```python
from build123d import *

# Parameters (mm, degrees)
ESQUISSE1_W                 = 200
ESQUISSE1_H                 = 200
BOSS_EXTRU_PAROIE_DEPTH     = 4
BOSS_EXTRU_BORDS_DEPTH      = 8
BOSS_EXTRU_GLISSIERES_DEPTH = 4
CONG_1_R                    = 1
ESQUISSE8_W                 = 1.8
ESQUISSE8_H                 = 180
ENL_V_MAT_EXTRU_6_DEPTH     = 9
ESQUISSE5_R                 = 1.6
ENL_V_MAT_EXTRU_2_DEPTH     = 10
ESQUISSE6_R                 = 1.6
ENL_V_MAT_EXTRU_3_DEPTH     = 10
ESQUISSE7_R                 = 1.6
ENL_V_MAT_EXTRU_4_DEPTH     = 10
ESQUISSE10_R                = 1.6
ENL_V_MAT_EXTRU_8_DEPTH     = 10
ESQUISSE11_W                = 113.303164178
ESQUISSE11_H                = 6
ENL_V_MAT_EXTRU_9_DEPTH     = 6
ESQUISSE9_R                 = 1.6
ENL_V_MAT_EXTRU_10_DEPTH    = 10


with BuildPart() as part:
    # Esquisse1 → Boss.-Extru. Paroie (new body)
    with BuildSketch(Plane.XY):
        with Locations((100, 100)):
            Rectangle(ESQUISSE1_W, ESQUISSE1_H)
    extrude(amount=BOSS_EXTRU_PAROIE_DEPTH)

    # Esquisse4 → Boss.-Extru. Bords (add)
    with BuildSketch(Plane.XY.offset(4)):
        Polygon((3, 3), (9, 3), (9, 184), (191, 184), (191, 3), (197, 3), (197, 197), (191, 197), (191, 190), (9, 190), (9, 197), (3, 197), align=None)
    extrude(amount=BOSS_EXTRU_BORDS_DEPTH)

    # Esquisse2 → Boss.-Extru. Glissieres (add)
    with BuildSketch(Plane.XY.offset(4)):
        with BuildLine():
            Line((47, 170), (53, 170))
            ThreePointArc((53, 170), (54.414213562, 169.414213562), (55, 168))
            Line((55, 168), (55, 32))
            ThreePointArc((55, 32), (54.414213562, 30.585786438), (53, 30))
            Line((53, 30), (47, 30))
            ThreePointArc((47, 30), (45.585786438, 30.585786438), (45, 32))
            Line((45, 32), (45, 168))
            ThreePointArc((45, 168), (45.585786438, 169.414213562), (47, 170))
        make_face()
        with BuildLine():
            Line((97, 170), (103, 170))
            ThreePointArc((103, 170), (104.414213562, 169.414213562), (105, 168))
            Line((105, 168), (105, 32))
            ThreePointArc((105, 32), (104.414213562, 30.585786438), (103, 30))
            Line((103, 30), (97, 30))
            ThreePointArc((97, 30), (95.585786438, 30.585786438), (95, 32))
            Line((95, 32), (95, 168))
            ThreePointArc((95, 168), (95.585786438, 169.414213562), (97, 170))
        make_face()
        with BuildLine():
            Line((147, 170), (153, 170))
            ThreePointArc((153, 170), (154.414213562, 169.414213562), (155, 168))
            Line((155, 168), (155, 32))
            ThreePointArc((155, 32), (154.414213562, 30.585786438), (153, 30))
            Line((153, 30), (147, 30))
            ThreePointArc((147, 30), (145.585786438, 30.585786438), (145, 32))
            Line((145, 32), (145, 168))
            ThreePointArc((145, 168), (145.585786438, 169.414213562), (147, 170))
        make_face()
    extrude(amount=BOSS_EXTRU_GLISSIERES_DEPTH)

    # Congé1
    cong_1_edges = [part.edges().sort_by_distance(p)[0] for p in [
        (200, 100, 4),
        (100, 200, 4),
        (0, 100, 4),
        (100, 0, 4),
    ]]
    fillet(cong_1_edges, radius=CONG_1_R)

    # Esquisse8 → Enlèv. mat.-Extru.6 (cut, through all)
    with BuildSketch(Plane.XY.offset(4)):
        with Locations((100, 85)):
            Rectangle(ESQUISSE8_W, ESQUISSE8_H)
        with Locations((150, 85)):
            Rectangle(ESQUISSE8_W, ESQUISSE8_H)
        with Locations((50, 85)):
            Rectangle(ESQUISSE8_W, ESQUISSE8_H)
    extrude(amount=ENL_V_MAT_EXTRU_6_DEPTH, mode=Mode.SUBTRACT)

    # Esquisse5 → Enlèv. mat.-Extru.2 (cut)
    with BuildSketch(Plane.ZY.offset(-3)):
        with Locations((8, 180)):
            Circle(ESQUISSE5_R)
        with Locations((8, 20)):
            Circle(ESQUISSE5_R)
    extrude(amount=-ENL_V_MAT_EXTRU_2_DEPTH, mode=Mode.SUBTRACT)

    # Esquisse6 → Enlèv. mat.-Extru.3 (cut)
    with BuildSketch(Plane(origin=(197, 0, 0), x_dir=(0, 0, -1), z_dir=(1, 0, 0))):
        with Locations((-8, 180)):
            Circle(ESQUISSE6_R)
        with Locations((-8, 20)):
            Circle(ESQUISSE6_R)
    extrude(amount=-ENL_V_MAT_EXTRU_3_DEPTH, mode=Mode.SUBTRACT)

    # Esquisse7 → Enlèv. mat.-Extru.4 (cut)
    with BuildSketch(Plane.XZ.offset(-184)):
        with Locations((35, 8)):
            Circle(ESQUISSE7_R)
        with Locations((165, 8)):
            Circle(ESQUISSE7_R)
    extrude(amount=-ENL_V_MAT_EXTRU_4_DEPTH, mode=Mode.SUBTRACT)

    # Esquisse10 → Enlèv. mat.-Extru.8 (cut)
    with BuildSketch(Plane(origin=(0, 3, 0), x_dir=(-1, 0, 0), z_dir=(0, -1, 0))):
        with Locations((-194.2, -8)):
            Circle(ESQUISSE10_R)
        with Locations((-5.8, -8)):
            Circle(ESQUISSE10_R)
    extrude(amount=-ENL_V_MAT_EXTRU_8_DEPTH, mode=Mode.SUBTRACT)

    # Esquisse11 → Enlèv. mat.-Extru.9 (cut)
    with BuildSketch(Plane.XY.offset(12)):
        with Locations((100.248809194, 187)):
            Rectangle(ESQUISSE11_W, ESQUISSE11_H)
    extrude(amount=-ENL_V_MAT_EXTRU_9_DEPTH, mode=Mode.SUBTRACT)

    # Esquisse9 → Enlèv. mat.-Extru.10 (cut)
    with BuildSketch(Plane(origin=(0, 197, 0), x_dir=(1, 0, 0), z_dir=(0, 1, 0))):
        with Locations((194.2, -8)):
            Circle(ESQUISSE9_R)
        with Locations((5.8, -8)):
            Circle(ESQUISSE9_R)
    extrude(amount=-ENL_V_MAT_EXTRU_10_DEPTH, mode=Mode.SUBTRACT)


solid = part.part
```
Geometry check sheet. Reference: the model listing, model coordinates, mm. A direction names the side the tool comes from. Round coordinates to 2 decimals unless told otherwise and drop trailing zeros. Loops run counter-clockwise (first coordinate to the right, second up) from the corner with the lowest first, then second, coordinate; pieces in that order, holes last. Notation, with made-up numbers: (3, -29.5) - (57, -29.5) arc R32 cw to (57, 2.5) - close; hole circle Ø9 at (-2.75, 29). An arc over 180 degrees is marked (long way). Use a Markdown table: item, result.
Q1. Cross-section at B-B on x = 88. Record the cut outline in (y, z).
Solutions:
| item | result |
|---|---|
| outline | (0, 0) - (200, 0) - (200, 3) arc R1 ccw to (199, 4) - (190, 4) - (190, 6) - (184, 6) - (184, 4) - (1, 4) arc R1 ccw to (0, 3) - close |
Q2. Cross-section at A-A on y = 173. Record the cut outline in (x, z).
Solutions:
| item | result |
|---|---|
| outline | (0, 0) - (200, 0) - (200, 3) arc R1 ccw to (199, 4) - (197, 4) - (197, 12) - (191, 12) - (191, 4) - (9, 4) - (9, 12) - (3, 12) - (3, 4) - (1, 4) arc R1 ccw to (0, 3) - close |
Q3. Go/stop test with flat-tipped pins: P1, Ø1.2, axis at y = 133.5, z = 6.5, coming from the +X side; P2, Ø12, axis at x = 64.5, y = 111, coming from the +Z side; P3, Ø5, axis at y = 188.5, z = 8, coming from the -X side; P4, Ø1, axis at x = 79, z = 1.5, coming from the -Y side. Record where each tip stops, or that it passes through.
Solutions:
| item | result |
|---|---|
| P1 | stops at x = 197 |
| P2 | stops at z = 4 |
| P3 | stops at x = 3 |
| P4 | stops at y = 0 |
Q4. Material ranges on line 1 (Y direction, x = 4.4, z = 8); line 2 (X direction, y = 15.5, z = 8.25); line 3 (Y direction, x = 99, z = 5), recorded low to high.
Solutions:
| item | result |
|---|---|
| line 1 | y = 13 to 18.4, 21.6 to 178.4, 181.6 to 187 |
| line 2 | x = 3 to 9, 191 to 197 |
| line 3 | y = 30 to 170, 184 to 190 |
Q5. Draft check along X on faces 1 (the flat face through (7.4, 197, 8.8)), 2 (the flat face through (197, 99, 8)), 3 (the flat face through (121, 79, 4)), 4 (the flat face through (191, 194, 8)). Enter one of: released by +X, released by -X, zero draft, split by the parting line, or undercut.
Solutions:
| item | result |
|---|---|
| face 1 | zero draft |
| face 2 | released by +X |
| face 3 | undercut |
| face 4 | undercut |
Q6. Access from +Z, -Z, +X, -X, +Y, -Y to the whole of each face (thin tool, end or side, straight path). Record for faces 5 (the flat face through (192.71, 197, 7.06)), 6 (the flat face through (9, 193, 8)), 7 (the flat face through (7.29, 3, 7.06)), 8 (the flat face through (191, 95, 8)), 9 (the flat face through (156.9, 187, 9)).
Solutions:
| item | result |
|---|---|
| face 5 | +Z, +X, -X, +Y |
| face 6 | +Z, +Y |
| face 7 | +Z, +X, -X, -Y |
| face 8 | +Z, -Y |
| face 9 | +Z, +Y, -Y |
